from build123d import *

# Parameters (mm, degrees)
SKETCH_1_R               = 15
SKETCH_1_R_2             = 10.25
EXTRUDE_1_DEPTH          = 150
CUT_EXTRUDE_1_DEPTH      = 154.703965854
CUT_EXTRUDE_1_DEPTH_BACK = 154.703965854
SKETCH_2_R               = 1.5
SKETCH_3_R               = 22.14266171
CUT_EXTRUDE_2_DEPTH      = 80
SKETCH_5_W               = 6
SKETCH_5_H               = 5.980913868
CUT_EXTRUDE_3_DEPTH      = 80


with BuildPart() as part:
    # 스케치1 → 보스-돌출1 (new body)
    with BuildSketch(Plane(origin=(0, 0, 0), x_dir=(1, 0, 0), z_dir=(0, 1, 0))):
        with Locations(Location((0, 0, 0), (0, 0, 270))):
            Circle(SKETCH_1_R)
        with Locations(Location((0, 0, 0), (0, 0, 270))):
            Circle(SKETCH_1_R_2, mode=Mode.SUBTRACT)
    extrude(amount=EXTRUDE_1_DEPTH)

    # 스케치2 → 컷-돌출1 (cut, two sides: drawn at the far end of the back side and taken through both)
    with BuildSketch(Plane(origin=(0, 0, -14.998485281), x_dir=(-1, 0, 0), z_dir=(0, 0, -1)).offset(-CUT_EXTRUDE_1_DEPTH_BACK)):
        with Locations(Location((0, 11.805761924, 0), (0, 0, 90))):
            Circle(SKETCH_2_R)
        with Locations(Location((0, 21.207864132, 0), (0, 0, 90))):
            Circle(SKETCH_2_R)
        with Locations(Location((0, 36.207864132, 0), (0, 0, 90))):
            Circle(SKETCH_2_R)
        with Locations(Location((0, 48.906437248, 0), (0, 0, 90))):
            Circle(SKETCH_2_R)
        with Locations(Location((0, 56.868147497, 0), (0, 0, 90))):
            Circle(SKETCH_2_R)
        with Locations(Location((0, 64.829857746, 0), (0, 0, 90))):
            Circle(SKETCH_2_R)
        with Locations(Location((0, 77.054405077, 0), (0, 0, 90))):
            Circle(SKETCH_2_R)
        with Locations(Location((0, 91.899672592, 0), (0, 0, 90))):
            Circle(SKETCH_2_R)
        with Locations(Location((0, 106.761531723, 0), (0, 0, 90))):
            Circle(SKETCH_2_R)
        with Locations(Location((0, 122.331098432, 0), (0, 0, 90))):
            Circle(SKETCH_2_R)
        with Locations(Location((0, 136.839103775, 0), (0, 0, 90))):
            Circle(SKETCH_2_R)
    extrude(amount=CUT_EXTRUDE_1_DEPTH + CUT_EXTRUDE_1_DEPTH_BACK, mode=Mode.SUBTRACT)

    # 스케치3 → 컷-돌출2 (cut)
    with BuildSketch(Plane(origin=(0, 150, 0), x_dir=(1, 0, 0), z_dir=(0, 1, 0))):
        Circle(SKETCH_3_R)
    extrude(amount=-CUT_EXTRUDE_2_DEPTH, mode=Mode.SUBTRACT)

    # 스케치5 → 컷-돌출3 (cut)
    with BuildSketch(Plane.XZ):
        with Locations((0, 12.107840203)):
            Rectangle(SKETCH_5_W, SKETCH_5_H)
    extrude(amount=-CUT_EXTRUDE_3_DEPTH, mode=Mode.SUBTRACT)


solid = part.part
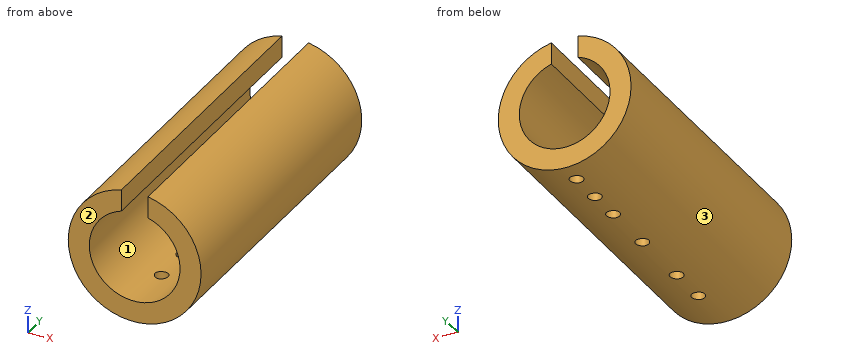
Design review of the part built by this model. Coordinates are the model's own, in mm. Face numbers are marked on the shaded views. Give positions to 0.01 mm unless a question says otherwise; leave off trailing zeros. Loops run counter-clockwise (first coordinate to the right, second up) from the corner with the lowest first, then second, coordinate; pieces in that order, holes last. Notation, with made-up numbers: M 77,-36 L 127,-36 A24 ccw 127,-5 Z; hole C 12.5,-39.5 d11. An arc over 180 degrees is marked long. Answer as a JSON object with one key per item and string values.
Item 1: We need section C-C (y = 65.5). State the section outline as (x, z) points, and give its area (3 significant figures).
Output values:
{"outline": "M -3,9.8 L -3,14.7 A15 ccw -1.34,-14.94 L -1.34,-10.16 A10.25 cw Z; M 1.34,-14.94 A15 ccw 3,14.7 L 3,9.8 A10.25 cw 1.34,-10.16 Z", "area": "335 mm2"}
Item 2: For P1, Ø5, axis at x = 0, y = 56.87, coming from the +Z side; P2, Ø12, axis at x = -6.5, z = -10, coming from the -Y side; P3, Ø5.5, axis at y = 26, z = 11, coming from the -X side; P4, Ø1.5, axis at y = 13.5, z = 2.5, coming from the -X side, all flat-tipped, find the tip position at first contact; note any pin that passes through.
Output values:
{"P1": "stops at z = -9.94", "P2": "stops at y = 0", "P3": "stops at x = -12.53", "P4": "stops at x = -14.9"}
Item 3: Wall thickness on line 1 along X through (y, z) = (48.5, -2.25); line 2 along Z through (x, y) = (-5.5, 23.5); line 3 along X through (y, z) = (27, 12.5): over which ranges is each line inside the solid? List them lowest first.
Output values:
{"line 1": "x = -14.83 to -10, 10 to 14.83", "line 2": "z = -13.96 to -8.65, 8.65 to 13.96", "line 3": "x = -8.29 to -3, 3 to 8.29"}
Item 4: We need section B-B (z = 0). State the section outline as (x, y) points.
Output values:
{"outline": "M -15,0 L -10.25,0 L -10.25,70 L -15,70 Z; M 10.25,0 L 15,0 L 15,70 L 10.25,70 Z"}
Item 5: Mouldability with a two-part tool opening along Z and no side actions: class the marked faces 1, 2 and 3 as pulls with the +Z half, pulls with the -Z half, needs draft (parallel to the pull), parting line crosses it, or undercut.
Output values:
{"face 1": "undercut", "face 2": "needs draft", "face 3": "parting line crosses it"}
Item 6: We need section A-A (x = 0). State the section outline as (y, z) points.
Output values:
{"outline": "M 0,-15 L 10.31,-15 L 10.31,-10.25 L 0,-10.25 Z; M 13.31,-15 L 19.71,-15 L 19.71,-10.25 L 13.31,-10.25 Z; M 22.71,-15 L 34.71,-15 L 34.71,-10.25 L 22.71,-10.25 Z; M 37.71,-15 L 47.41,-15 L 47.41,-10.25 L 37.71,-10.25 Z; M 50.41,-15 L 55.37,-15 L 55.37,-10.25 L 50.41,-10.25 Z; M 58.37,-15 L 63.33,-15 L 63.33,-10.25 L 58.37,-10.25 Z; M 66.33,-15 L 70,-15 L 70,-10.25 L 66.33,-10.25 Z"}
Item 7: We need section D-D (x = -12.5). State the section outline as (y, z) points.
Output values:
{"outline": "M 0,-8.29 L 70,-8.29 L 70,8.29 L 0,8.29 Z"}
